```python
from build123d import *

# Parameters (mm, degrees)
EXTRUDE_1_DEPTH = 5
SKETCH_2_R      = 12.5
SKETCH_2_R_2    = 1.5
SKETCH_2_R_3    = 4
EXTRUDE_2_DEPTH = 5
SKETCH_3_W      = 10
SKETCH_3_H      = 5
EXTRUDE_3_DEPTH = 5


with BuildPart() as part:
    # 草图1 → 凸台-拉伸1 (new body)
    with BuildSketch(Plane(origin=(0, 0, 0), x_dir=(1, 0, 0), z_dir=(0, 1, 0))):
        with BuildLine():
            ThreePointArc((15, 11.55), (0, 26.55), (-15, 11.55))
            Line((-15, 11.55), (-12.5, 11.55))
            ThreePointArc((-12.5, 11.55), (0, 24.05), (12.5, 11.55))
            Line((12.5, 11.55), (15, 11.55))
        make_face()
        with BuildLine():
            Line((-12.5, 11.55), (-15, 11.55))
            ThreePointArc((-15, 11.55), (0, -3.45), (15, 11.55))
            Line((15, 11.55), (12.5, 11.55))
            ThreePointArc((12.5, 11.55), (0, -0.95), (-12.5, 11.55))
        make_face()
        with BuildLine():
            ThreePointArc((15, 11.55), (0, 26.55), (-15, 11.55))
            Line((-15, 11.55), (-12.5, 11.55))
            ThreePointArc((-12.5, 11.55), (0, 24.05), (12.5, 11.55))
            Line((12.5, 11.55), (15, 11.55))
        make_face()
        with BuildLine():
            Line((-12.5, 11.55), (-15, 11.55))
            ThreePointArc((-15, 11.55), (0, -3.45), (15, 11.55))
            Line((15, 11.55), (12.5, 11.55))
            ThreePointArc((12.5, 11.55), (0, -0.95), (-12.5, 11.55))
        make_face()
        with BuildLine():
            Line((-15, 11.55), (-15, -11.55))
            Line((-15, -11.55), (15, -11.55))
            Line((15, -11.55), (15, 11.55))
            ThreePointArc((15, 11.55), (0, -3.45), (-15, 11.55))
        make_face()
    extrude(amount=EXTRUDE_1_DEPTH)

    # 草图2 → 凸台-拉伸2 (add)
    with BuildSketch(Plane(origin=(0, 5, 0), x_dir=(1, 0, 0), z_dir=(0, 1, 0))):
        with Locations((0, 11.55)):
            Circle(SKETCH_2_R)
        with Locations((-8.5, 11.55)):
            Circle(SKETCH_2_R_2, mode=Mode.SUBTRACT)
        with Locations((8.5, 11.55)):
            Circle(SKETCH_2_R_2, mode=Mode.SUBTRACT)
        with Locations((0, 11.55)):
            Circle(SKETCH_2_R_3, mode=Mode.SUBTRACT)
    extrude(amount=-EXTRUDE_2_DEPTH)

    # 草图3 → 凸台-拉伸3 (add)
    with BuildSketch(Plane(origin=(0, 5, 0), x_dir=(1, 0, 0), z_dir=(0, 1, 0))):
        with Locations((0, -14.05)):
            Rectangle(SKETCH_3_W, SKETCH_3_H)
    extrude(amount=-EXTRUDE_3_DEPTH)


solid = part.part
```
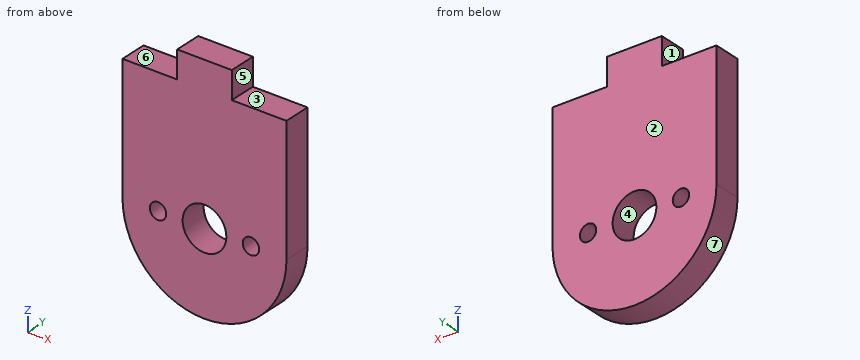
Part model, mm, in its own coordinate system. Face numbers are marked on the shaded views. A direction names the side the tool comes from. Round coordinates to 2 decimals unless told otherwise and drop trailing zeros. Loops run counter-clockwise (first coordinate to the right, second up) from the corner with the lowest first, then second, coordinate; pieces in that order, holes last.
Item 1: 3-axis set-ups, long thin cutter, end or side, ignore diameter. For the marked faces 1, 2 and 3: which of +Z, -Z, +X, -X, +Y, -Y reach the whole face in a straight line?
Item 2: Drill centre lines: line 1 (X direction, y = 3.75, z = -11.55); line 2 (Z direction, x = 0, y = 4); line 3 (Z direction, x = 9, y = 4.3). Where is each one in solid material? Low to high.
Item 3: Cut at D-D, the plane x = 8. Give the cut face in (y, z).
Item 4: Mould opens along Z. For the marked faces 4, 5, 6 and 7 say: +Z half, -Z half, draft (parallel to the pull), parting line (faces both ways), or undercut.
Item 5: Drop flat-ended pins along their axis: P1, Ø1.5, axis at x = -12, y = 2, coming from the +Z side; P2, Ø4, axis at x = 8.5, z = -11.55, coming from the -Y side. Give the stop position or say it passes through.
Item 6: Cut at A-A, the plane x = 0. Give the cut face in (y, z).
Item 7: Cut at C-C, the plane z = 13. Give the cut face in (x, y), then the cut area to 3 significant figures.
Item 8: Cut at B-B, the plane y = 4.35. Give the cut face in (x, z), then the cut area to 3 significant figures.
A:
1. face 1: +Z, -X, +Y, -Y
1. face 2: +Z, -Z, +X, -X, +Y
1. face 3: +Z, +X, +Y, -Y
2. line 1: x = -15 to -10, -7 to -4, 4 to 7, 10 to 15
2. line 2: z = -26.55 to -15.55, -7.55 to 16.55
2. line 3: z = -23.55 to -12.96, -10.14 to 11.55
3. outline: (0, -24.24) - (5, -24.24) - (5, -12.96) - (0, -12.96) - close; (0, -10.14) - (5, -10.14) - (5, 11.55) - (0, 11.55) - close
4. face 4: undercut
4. face 5: draft
4. face 6: +Z half
4. face 7: -Z half
5. P1: stops at z = 11.55
5. P2: stops at y = 0
6. outline: (0, -26.55) - (5, -26.55) - (5, -15.55) - (0, -15.55) - close; (0, -7.55) - (5, -7.55) - (5, 16.55) - (0, 16.55) - close
7. outline: (-5, 0) - (5, 0) - (5, 5) - (-5, 5) - close
7. area: 50.0 mm2
8. outline: (-15, -11.55) arc R15 ccw to (15, -11.55) - (15, 11.55) - (5, 11.55) - (5, 16.55) - (-5, 16.55) - (-5, 11.55) - (-15, 11.55) - close; hole circle Ø3 at (-8.5, -11.55); hole circle Ø8 at (0, -11.55); hole circle Ø3 at (8.5, -11.55)
8. area: 1,030 mm2
